Verification items for the finished model (mm, model axes). Give positions to 0.01 mm unless a question says otherwise; leave off trailing zeros. Order: outer loops, then holes, each group sorted by start corner. A loop starts at its lowest first (then second) coordinate and runs counter-clockwise, first axis right, second up. Notation, with made-up numbers: (76, 24.5) - (93, 24.5) arc R36 cw to (93, 60.5) - close; hole circle Ø5 at (73, -1). An arc over 180 degrees is marked (long way). Answer as a JSON object with one key per item and string values. Group by question number.
(1) Depth check by flat-ended pin: pin 1 Ø11 at (x, z) = (0, 0) entering from +Y; pin 2 Ø10 at (x, y) = (3, -3) entering from -Z; pin 3 Ø4 at (y, z) = (0, -3.5) entering from -X; pin 4 Ø4 at (x, y) = (-10, -0.5) entering from +Z. Enter the tip coordinate at first touch or a pass-through.
(2) Thickness scan on line 1 (X direction, y = -0.75, z = -0.25); line 2 (Z direction, x = 0, y = 1.25); line 3 (Z direction, x = 0, y = -3). Record the ranges inside material, lowest first.
(3) Section check A-A (z = 0). Record the boundary of the cut face in (x, y), then the cut area to 3 significant figures.
(4) Mould release check, pull along Z, two halves, no side actions. Record for faces 1 (the face through (10, 0, -7)), 2 (the face through (11.207, -3.944, 3.529)), 3 (the face through (6, 4, 0)): +Z half, -Z half, draft (parallel to the pull), parting line (faces both ways), or undercut.
(5) Section check C-C (y = 4.5). Record the boundary of the cut face in (x, z).
(6) Section check D-D (z = -10.5). Record the boundary of the cut face in (x, y), then the cut area to 3 significant figures.
(7) Section check B-B (x = 0). Record the boundary of the cut face in (y, z).
```python
from build123d import *

# Parameters (mm, degrees)
F0_R     = 11.75
F1_DEPTH = 8
F2_R     = 13
F3_DEPTH = 15
F4_R     = 6
F5_DEPTH = 25


with BuildPart() as f1:
    # F0 (on Front) → F1 (new body)
    with BuildSketch(Plane.XZ):
        Circle(F0_R)
    extrude(amount=F1_DEPTH)

    # F2 (on face) → F3 (join)
    with BuildSketch(Plane(origin=(0, 0, 0), x_dir=(-1, 0, 0), z_dir=(0, 1, 0))):
        Circle(F2_R)
    extrude(amount=F3_DEPTH)

    # F4 (on face) → F5 (cut)
    with BuildSketch(Plane(origin=(0, 15, 0), x_dir=(-1, 0, 0), z_dir=(0, 1, 0))):
        Circle(F4_R)
    extrude(amount=-F5_DEPTH, mode=Mode.SUBTRACT)


solid = f1.part
```
Solutions:
{
 "1": {"pin 1": "passes through", "pin 2": "stops at z = -13", "pin 3": "stops at x = -12.91", "pin 4": "stops at z = 10.2"},
 "2": {"line 1": "x = -11.75 to -5.99, 5.99 to 11.75", "line 2": "z = -13 to -6, 6 to 13", "line 3": "z = -11.75 to -6, 6 to 11.75"},
 "3": {"outline": "(-13, 0) - (-11.75, 0) - (-11.75, -8) - (-6, -8) - (-6, 15) - (-13, 15) - close; (6, -8) - (11.75, -8) - (11.75, 0) - (13, 0) - (13, 15) - (6, 15) - close", "area": "302 mm2"},
 "4": {"face 1": "draft", "face 2": "parting line", "face 3": "undercut"},
 "5": {"outline": "circle Ø26 at (0, 0); hole circle Ø12 at (0, 0)"},
 "6": {"outline": "(-7.66, 0) - (-5.27, 0) - (-5.27, -8) - (5.27, -8) - (5.27, 0) - (7.66, 0) - (7.66, 15) - (-7.66, 15) - close", "area": "314 mm2"},
 "7": {"outline": "(-8, -11.75) - (0, -11.75) - (0, -13) - (15, -13) - (15, -6) - (-8, -6) - close; (-8, 6) - (15, 6) - (15, 13) - (0, 13) - (0, 11.75) - (-8, 11.75) - close"}
}
